Print and shaded views of the part. All mm, measured from the part's lowest x, y and z. A direction names the side the tool comes from. Round coordinates to 2 decimals unless told otherwise and drop trailing zeros. Order: outer loops, then holes, each group sorted by start corner. A loop starts at its lowest first (then second) coordinate and runs counter-clockwise, first axis right, second up. Notation, with made-up numbers: (62, 78) - (102, 78) arc R18 ccw to (102, 87) - close; hole circle Ø9 at (89.25, 35). An arc over 180 degrees is marked (long way). Return JSON: item names as keys, results as strings. Group by question number.
Item 1: Saw through at C-C on y = 29. List the corners of the cut face in (x, z), and give its area (3 significant figures).
Item 2: Saw through at A-A on z = 7. List the corners of the cut face in (x, y).
Item 3: Tool access for the marked faces 5, 6, 7, 8 and 9: list every direction of +Z, -Z, +X, -X, +Y, -Y with a clear straight run to the whole face (end or side of a thin tool).
Item 4: Two-plate mould, pull along X, no slides. Class the marked faces 1, 2, 3 and 4: released by +X, released by -X, zero draft, split by the parting line, or undercut.
Item 5: Saw through at B-B on x = 132. List the corners of the cut face in (y, z), and give its area (3 significant figures).
Item 6: Saw through at D-D on z = 16.5. List the corners of the cut face in (x, y).
Item 7: Drop flat-ended pins along their axis: pin 1 (4 mm diameter, centred on y = 18.5, z = 14, fed in from +X); pin 2 (20.5 mm diameter, centred on x = 7, y = 46, fed in from +Z); pin 3 (21 mm diameter, centred on y = 51.5, z = 8.5, fed in from +X). Give the stop position or say it passes through.
Item 8: Probe probe 1 along X at (y, z) = (39.5, 3); probe 2 along X at (y, z) = (63, 18); probe 3 along X at (y, z) = (70.5, 39). List the from-to ranges inside material, lowest first.
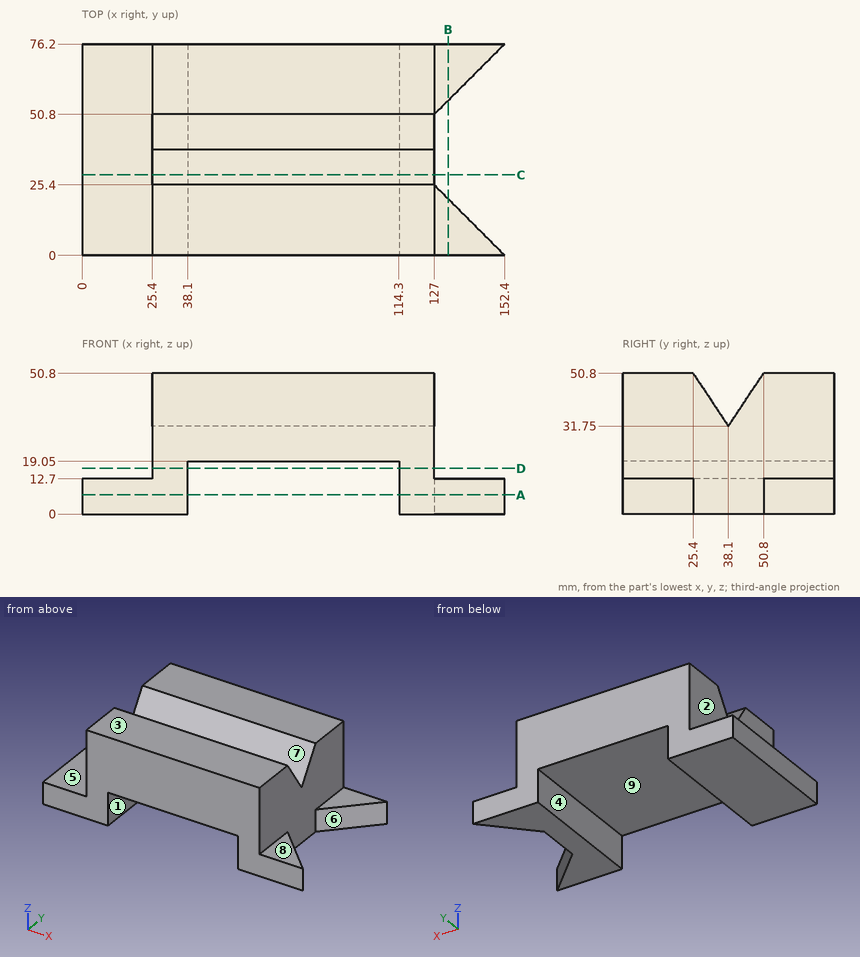
Filled in:
{
 "1": {"outline": "(0, 0) - (38.1, 0) - (38.1, 19.05) - (114.3, 19.05) - (114.3, 0) - (127, 0) - (127, 45.4) - (25.4, 45.4) - (25.4, 12.7) - (0, 12.7) - close", "area": "3,480 mm^2"},
 "2": {"outline": "(0, 0) - (38.1, 0) - (38.1, 76.2) - (0, 76.2) - close; (114.3, 0) - (152.4, 0) - (127, 25.4) - (127, 50.8) - (152.4, 76.2) - (114.3, 76.2) - close"},
 "3": {"face 5": "+Z, -X, +Y, -Y", "face 6": "+Z, -Z, +X", "face 7": "+Z, +X, -X", "face 8": "+Z, +X, +Y, -Y", "face 9": "-Z, +Y, -Y"},
 "4": {"face 1": "undercut", "face 2": "released by -X", "face 3": "zero draft", "face 4": "undercut"},
 "5": {"outline": "(0, 0) - (20.4, 0) - (20.4, 12.7) - (0, 12.7) - close; (55.8, 0) - (76.2, 0) - (76.2, 12.7) - (55.8, 12.7) - close", "area": "518 mm^2"},
 "6": {"outline": "(25.4, 0) - (38.1, 0) - (38.1, 76.2) - (25.4, 76.2) - close; (114.3, 0) - (127, 0) - (127, 76.2) - (114.3, 76.2) - close"},
 "7": {"pin 1": "stops at x = 135.42", "pin 2": "stops at z = 12.7", "pin 3": "stops at x = 138.2"},
 "8": {"probe 1": "x = 0 to 38.1, 114.3 to 127", "probe 2": "x = 25.4 to 38.1, 114.3 to 127", "probe 3": "x = 25.4 to 127"}
}
